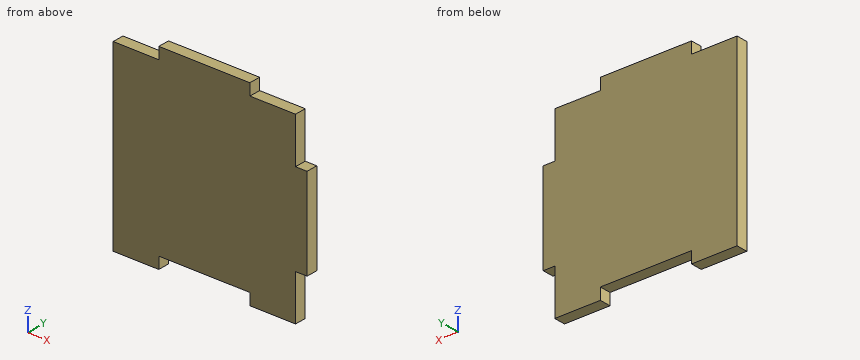
from build123d import *

# Parameters (mm, degrees)
SKETCH1_W           = 50
SKETCH1_H           = 50
BOSS_EXTRUDE1_DEPTH = 3.175
SKETCH3_W           = 3.175
SKETCH3_H           = 25
SKETCH3_W_2         = 25
SKETCH3_H_2         = 3.175
BOSS_EXTRUDE3_DEPTH = 3.175
SKETCH4_W           = 25
SKETCH4_H           = 3.175
CUT_EXTRUDE1_DEPTH  = 3.175


with BuildPart() as part:
    # Sketch1 → Boss-Extrude1 (new body)
    with BuildSketch(Plane(origin=(0, 0, 0), x_dir=(1, 0, 0), z_dir=(0, 1, 0))):
        Rectangle(SKETCH1_W, SKETCH1_H)
    extrude(amount=BOSS_EXTRUDE1_DEPTH)

    # Sketch3 → Boss-Extrude3 (add)
    with BuildSketch(Plane(origin=(0, 3.175, 0), x_dir=(1, 0, 0), z_dir=(0, 1, 0))):
        with Locations((26.5875, 0)):
            Rectangle(SKETCH3_W, SKETCH3_H)
        with Locations((0, -26.5875)):
            Rectangle(SKETCH3_W_2, SKETCH3_H_2)
    extrude(amount=-BOSS_EXTRUDE3_DEPTH)

    # Sketch4 → Cut-Extrude1 (cut)
    with BuildSketch(Plane(origin=(0, 3.175, 0), x_dir=(1, 0, 0), z_dir=(0, 1, 0))):
        with Locations((0, 23.4125)):
            Rectangle(SKETCH4_W, SKETCH4_H)
    extrude(amount=-CUT_EXTRUDE1_DEPTH, mode=Mode.SUBTRACT)


solid = part.part
For this review, take the finished solid that the model builds, in its own axes (mm). Round coordinates to 2 decimals unless told otherwise and drop trailing zeros. Write each loop counter-clockwise with the first axis right and the second up, starting at its lowest first coordinate (ties: lowest second). Pieces come first, ordered by that corner, then holes. Notation, with made-up numbers: (83, 35) - (90, 35) arc R15 ccw to (90, 52) - close; hole circle Ø9 at (12, 17.25). An arc over 180 degrees is marked (long way). Write item = value, one per line. Start each with the question number.
1. Consider section C-C on x = 7. State the section outline as (y, z) points (3 decimals).
2. Consider section B-B on z = 21. State the section outline as (x, y) points (3 decimals).
3. Consider section A-A on y = 2.3. State the section outline as (x, z) points (3 decimals).
4. For pin 1 Ø1.6 at (y, z) = (2, -23) entering from +X; pin 2 Ø1.6 at (x, y) = (26.5, 1) entering from -Z; pin 3 Ø1.6 at (y, z) = (2, 26) entering from +X, all flat-tipped, find the tip position at first contact; note any pin that passes through.
5. Wall thickness on L1, parallel to Z at x = -20.5, y = 0.2; L2, parallel to Z at x = -1, y = 1.55 (3 decimals): over which ranges is each line inside the solid? List them lowest first.
Evaluation:
q1.outline = (0, -21.825) - (3.175, -21.825) - (3.175, 28.175) - (0, 28.175) - close
q2.outline = (-25, 0) - (25, 0) - (25, 3.175) - (-25, 3.175) - close
q3.outline = (-25, -25) - (-12.5, -25) - (-12.5, -21.825) - (12.5, -21.825) - (12.5, -25) - (25, -25) - (25, -12.5) - (28.175, -12.5) - (28.175, 12.5) - (25, 12.5) - (25, 25) - (12.5, 25) - (12.5, 28.175) - (-12.5, 28.175) - (-12.5, 25) - (-25, 25) - close
q4.pin_1 = 25
q4.pin_2 = -12.5
q4.pin_3 = 12.5
q5.L1 = -25 to 25
q5.L2 = -21.825 to 28.175
